CAD build for the part. Positions are in the model's coordinates, mm. Give positions to 0.01 mm unless a question says otherwise; leave off trailing zeros. Loops run counter-clockwise (first coordinate to the right, second up) from the corner with the lowest first, then second, coordinate; pieces in that order, holes last. Notation, with made-up numbers: (70, -7) - (115, -7) arc R19 cw to (115, 23) - close; hole circle Ø5 at (29, 86). An arc over 180 degrees is marked (long way). Return JSON: item names as keys, results as strings.
Autodesk Inventor part; units mm, degrees
ref_plane "YZ Plane" through (0, 0, 0) normal (1, 0, 0) x (0, 1, 0)
ref_plane "XZ Plane" through (0, 0, 0) normal (0, 1, 0) x (-1, 0, 0)
ref_plane "XY Plane" through (0, 0, 0) normal (0, 0, 1) x (1, 0, 0)
sketch "Sketch1" plane through (0, 0, 0) normal (0, 0, 1) x (1, 0, 0)
  line L0 (0, 0) -> (5.461, 0)
  line L1 (5.461, 0) -> (5.461, 39.8272)
  line L2 (5.461, 39.8272) -> (0, 39.8272)
  line L3 (0, 39.8272) -> (0, 0)
  dimension "d0" = 5.461
  dimension "d1" = 39.8272
extrude "Extrusion1" add sketch "Sketch1" along normal blind 609.6
sketch "Sketch2" plane through (0, 0, 609.6) normal (0, 0, 1) x (1, 0, 0)
  line L0 (5.461, 0) -> (5.461, 39.8272)
  line L1 (5.461, 0) -> (4.191, 0) construction
  line L2 (0, 0) -> (5.461, 0)
  line L3 (4.191, 0) -> (9.1821, 0) construction
  circle A0 centre (9.1821, 0) radius 4.9911
  line L4 (5.461, 19.9136) -> (0, 19.9136) construction
  line L5 (0, 39.8272) -> (0, 0) construction
  line L6 (5.461, 39.8272) -> (4.191, 39.8272) construction
  circle A1 centre (9.1821, 39.8272) radius 4.9911
  dimension "d4" = 1.27
  dimension "d5" = 4.9911
extrude "Extrusion2" add sketch "Sketch2" against normal blind 609.6
properties part number "Linear Guide Rail Temporary"
1. Cut at B-B, the plane z = 341. Write the cut outline in (x, y).
Values follow:
{"outline": "(0, 0) - (4.19, 0) arc R4.99 ccw (long way) to (5.46, 3.33) - (5.46, 36.5) arc R4.99 ccw (long way) to (4.19, 39.83) - (0, 39.83) - close"}
2. Drill centre lines: probe 1 along Y at (x, z) = (10.25, 206); probe 2 along Y at (x, z) = (9.75, 83.5); probe 3 along X at (y, z) = (15, 571.5). Where is each one in solid material? Low to high.
Values follow:
{"probe 1": "y = -4.88 to 4.88, 34.95 to 44.7", "probe 2": "y = -4.96 to 4.96, 34.87 to 44.79", "probe 3": "x = 0 to 5.46"}
3. Cut at A-A, the plane x = 10.25. Write the cut outline in (y, z).
Values follow:
{"outline": "(-4.88, 0) - (4.88, 0) - (4.88, 609.6) - (-4.88, 609.6) - close; (34.95, 0) - (44.7, 0) - (44.7, 609.6) - (34.95, 609.6) - close"}
4. Cut at C-C, the plane y = 29. Write the cut outline in (x, z).
Values follow:
{"outline": "(0, 0) - (5.46, 0) - (5.46, 609.6) - (0, 609.6) - close"}
5. Pull direction Y, two halves, no side cores. Call faces 1 (the face through (5, 20, 0)), 2 (the face through (13.911, 41.425, 309.067)): +Y half, -Y half, draft (parallel to the pull), parting line (faces both ways), or undercut.
Values follow:
{"face 1": "draft", "face 2": "undercut"}
6. Drop flat-ended pins along their axis: P1, Ø8, axis at x = 7.5, z = 338.5, coming from the +Y side; P2, Ø1.3, axis at x = 3, z = 241, coming from the -Y side; P3, Ø2, axis at x = 3, z = 153, coming from the +Y side; P4, Ø1, axis at x = 8, z = 92, coming from the -Y side. Give the stop position or say it passes through.
Values follow:
{"P1": "stops at y = 44.82", "P2": "stops at y = 0", "P3": "stops at y = 39.83", "P4": "stops at y = -4.94"}
